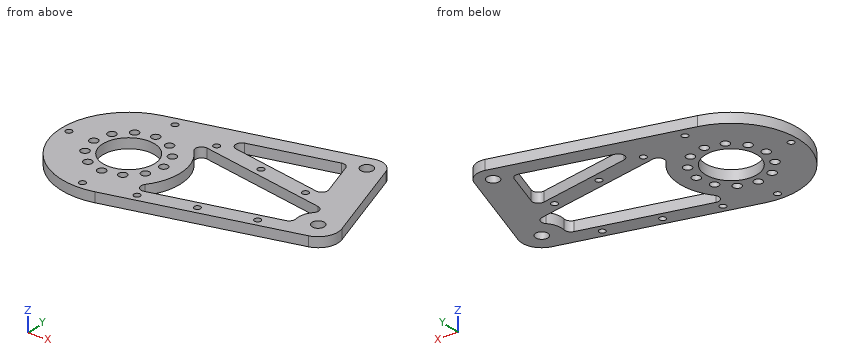
from build123d import *

# Parameters (mm, degrees)
SKETCH_1_R          = 3.1
SKETCH_1_R_2        = 13.1
SKETCH_1_R_3        = 1.6
EXTRUDE_1_DEPTH     = 5
SKETCH_3_R          = 2.1
CUT_EXTRUDE_1_DEPTH = 34
CUT_EXTRUDE_START   = -24
CUT_EXTRUDE_2_DEPTH = 24
FILLET_1_R          = 3
SKETCH_5_R          = 1.6
CUT_EXTRUDE_3_DEPTH = 24
CUT_EXTRUDE_4_DEPTH = 34
FILLET_2_R          = 3


with BuildPart() as part:
    # 草图1 → 凸台-拉伸1 (new body)
    with BuildSketch(Plane.XY):
        with BuildLine():
            Line((-103.589105886, 32.89722268), (-14.961918346, 56.036814298))
            ThreePointArc((-14.961918346, 56.036814298), (-9.057902271, 55.29071215), (-5.302552139, 50.674282835))
            Line((-5.302552139, 50.674282835), (9.548000145, 2.9724894))
            ThreePointArc((9.548000145, 2.9724894), (8.743053177, -4.853763606), (2.526315789, -9.675625485))
            Line((2.526315789, -9.675625485), (-86.410526316, -32.89712665))
            ThreePointArc((-86.410526316, -32.89712665), (-127.897174666, -8.589289785), (-103.589105886, 32.89722268))
        make_face()
        Circle(SKETCH_1_R, mode=Mode.SUBTRACT)
        with Locations((-95, 0)):
            Circle(SKETCH_1_R_2, mode=Mode.SUBTRACT)
        with Locations((-12.940952255, 48.296291314)):
            Circle(SKETCH_1_R, mode=Mode.SUBTRACT)
        with Locations((-95, 30)):
            Circle(SKETCH_1_R_3, mode=Mode.SUBTRACT)
        with Locations((-125, 0)):
            Circle(SKETCH_1_R_3, mode=Mode.SUBTRACT)
        with Locations((-95, -30)):
            Circle(SKETCH_1_R_3, mode=Mode.SUBTRACT)
    extrude(amount=EXTRUDE_1_DEPTH)

    # 草图3 → 切除-拉伸1 (cut)
    with BuildSketch(Plane.XY.offset(5)):
        with Locations((-95, 17.5)):
            Circle(SKETCH_3_R)
        with Locations((-86.25, 15.155444566)):
            Circle(SKETCH_3_R)
        with Locations((-79.844555434, 8.75)):
            Circle(SKETCH_3_R)
        with Locations((-77.5, 0)):
            Circle(SKETCH_3_R)
        with Locations((-79.844555434, -8.75)):
            Circle(SKETCH_3_R)
        with Locations((-86.25, -15.155444566)):
            Circle(SKETCH_3_R)
        with Locations((-95, -17.5)):
            Circle(SKETCH_3_R)
        with Locations((-103.75, -15.155444566)):
            Circle(SKETCH_3_R)
        with Locations((-110.155444566, -8.75)):
            Circle(SKETCH_3_R)
        with Locations((-112.5, 0)):
            Circle(SKETCH_3_R)
        with Locations((-110.155444566, 8.75)):
            Circle(SKETCH_3_R)
        with Locations((-103.75, 15.155444566)):
            Circle(SKETCH_3_R)
    extrude(amount=-CUT_EXTRUDE_1_DEPTH, mode=Mode.SUBTRACT)

    # 草图4 → 切除-拉伸2 (cut)
    with BuildSketch(Plane.XY.offset(5).offset(CUT_EXTRUDE_START)):
        with BuildLine():
            Line((-90.621052632, 25.628593796), (1.684210526, 9.85715146))
            ThreePointArc((1.684210526, 9.85715146), (-8.011191904, 5.985048394), (-8.974874995, -4.410398942))
            Line((-8.974874995, -4.410398942), (-88.431578947, -25.156626262))
            ThreePointArc((-88.431578947, -25.156626262), (-69.024129218, 1.119882624), (-90.621052632, 25.628593796))
        make_face()
    extrude(amount=CUT_EXTRUDE_2_DEPTH, mode=Mode.SUBTRACT)

    # 圆角1
    fillet_1_edges = [part.edges().sort_by_distance(p)[0] for p in [
        (-88.431578947, -25.156626262, 2.5),
        (-90.621052632, 25.628593796, 2.5),
        (1.684210526, 9.85715146, 2.5),
        (-8.974874995, -4.410398942, 2.5),
    ]]
    fillet(fillet_1_edges, radius=FILLET_1_R)

    # 草图5 → 切除-拉伸3 (cut)
    with BuildSketch(Plane.XY.offset(5)):
        with Locations((-71.551753536, -24.883386101)):
            Circle(SKETCH_5_R)
        with Locations((-46.395127275, -18.314965049)):
            Circle(SKETCH_5_R)
        with Locations((-21.238501013, -11.746543996)):
            Circle(SKETCH_5_R)
        with Locations((-71.274432107, 26.380963088)):
            Circle(SKETCH_5_R)
        with Locations((-45.645838312, 22.002015719)):
            Circle(SKETCH_5_R)
        with Locations((-20.017244516, 17.623068351)):
            Circle(SKETCH_5_R)
    extrude(amount=-CUT_EXTRUDE_3_DEPTH, mode=Mode.SUBTRACT)

    # 草图6 → 切除-拉伸4 (cut)
    with BuildSketch(Plane.XY.offset(5)):
        Polygon((-77.356433109, 31.478112128), (-20.689823209, 46.27314566), (-12.641453143, 20.420794919), align=None)
    extrude(amount=-CUT_EXTRUDE_4_DEPTH, mode=Mode.SUBTRACT)

    # 圆角2
    fillet_2_edges = [part.edges().sort_by_distance(p)[0] for p in [
        (-12.641453143, 20.420794919, 2.5),
        (-77.356433109, 31.478112128, 2.5),
        (-20.689823209, 46.27314566, 2.5),
    ]]
    fillet(fillet_2_edges, radius=FILLET_2_R)


solid = part.part
Work out the finished part from the listing and answer in its coordinate system (mm). Round coordinates to 2 decimals unless told otherwise and drop trailing zeros. Write each loop counter-clockwise with the first axis right and the second up, starting at its lowest first coordinate (ties: lowest second). Pieces come first, ordered by that corner, then holes. Notation, with made-up numbers: M -6,73.25 L 1,73.25 A33 ccw 1,102.25 Z; hole C 7,-17 d11. An arc over 180 degrees is marked long. Use a Markdown table: item, result.
1) The part is cut by section D-D on y = 40. Give the vertices of the cut face in (x, z), plus the area to 3 significant figures.
Taken from the geometry:
| item | result |
|---|---|
| outline | M -76.38,0 L -44.72,0 L -44.72,5 L -76.38,5 Z; M -18.74,0 L -1.98,0 L -1.98,5 L -18.74,5 Z |
| area | 242 mm2 |
2) The part is cut by section C-C on x = -95. Give the vertices of the cut face in (y, z), plus the area to 3 significant figures.
Taken from the geometry:
| item | result |
|---|---|
| outline | M -34,0 L -31.6,0 L -31.6,5 L -34,5 Z; M -28.4,0 L -19.6,0 L -19.6,5 L -28.4,5 Z; M -15.4,0 L -13.1,0 L -13.1,5 L -15.4,5 Z; M 13.1,0 L 15.4,0 L 15.4,5 L 13.1,5 Z; M 19.6,0 L 28.4,0 L 28.4,5 L 19.6,5 Z; M 31.6,0 L 35.14,0 L 35.14,5 L 31.6,5 Z |
| area | 141 mm2 |
3) Consider line 1 (Y direction, x = -61.5, z = 3.05); line 2 (Y direction, x = -49, z = 3.3); line 3 (Y direction, x = -45, z = 1.5). Determine where each line is inside the solid, lowest interval first. Write a range as [from, to].
Taken from the geometry:
| item | result |
|---|---|
| line 1 | y = [-26.39, -18.12], [20.65, 28.77], [35.62, 43.89] |
| line 2 | y = [-23.13, -14.86], [18.52, 26.63], [38.88, 47.15] |
| line 3 | y = [-22.08, -19.1], [-17.53, -13.82], [17.83, 20.54], [23.47, 25.95], [39.93, 48.19] |
4) The part is cut by section B-B on y = -30. Give the vertices of the cut face in (x, z).
Taken from the geometry:
| item | result |
|---|---|
| outline | M -111,0 L -96.6,0 L -96.6,5 L -111,5 Z; M -93.4,0 L -75.31,0 L -75.31,5 L -93.4,5 Z |
5) The part is cut by section A-A on x = -54. Give the vertices of the cut face in (y, z), plus the area to 3 significant figures.
Taken from the geometry:
| item | result |
|---|---|
| outline | M -24.43,0 L -16.17,0 L -16.17,5 L -24.43,5 Z; M 19.37,0 L 27.49,0 L 27.49,5 L 19.37,5 Z; M 37.58,0 L 45.84,0 L 45.84,5 L 37.58,5 Z |
| area | 123 mm2 |
6) Flat-ended cylindrical pins translate along their axes: pin 1 (1.5 mm diameter, centred on x = -31.5, z = 4, fed in from -Y); pin 2 (1.5 mm diameter, centred on x = -75, z = 2, fed in from -Y); pin 3 (3 mm diameter, centred on y = 11.5, z = 4, fed in from -X). Find the tip coordinate at first contact, or state that the pin passes through.
Taken from the geometry:
| item | result |
|---|---|
| pin 1 | stops at y = -18.76 |
| pin 2 | stops at y = -30.11 |
| pin 3 | stops at x = -127.5 |
